```python
from build123d import *

# Parameters (mm, degrees)
F0_W     = 112
F0_H     = 30
F0_R     = 4
F1_DEPTH = 3
F3_DEPTH = 25
F4_R     = 4
F5_DEPTH = 25


with BuildPart() as f1:
    # F0 (on Front) → F1 (new body)
    with BuildSketch(Plane.XZ):
        Rectangle(F0_W, F0_H)
        with Locations((-45.5, 8)):
            Circle(F0_R, mode=Mode.SUBTRACT)
    extrude(amount=F1_DEPTH)

    # F2 (on face) → F3 (cut)
    with BuildSketch(Plane.XZ.offset(3)):
        Polygon((-39, 5), (-39, 2), (-39, -1), (-32, -1), (-32, -8), (-29, -8), (-26, -8), (-26, -1), (-19, -1), (-19, 2), (-19, 5), (-26, 5), (-26, 12), (-29, 12), (-32, 12), (-32, 5), align=None)
    extrude(amount=-F3_DEPTH, mode=Mode.SUBTRACT)

    # F4 (on face) → F5 (cut)
    with BuildSketch(Plane.XZ.offset(3)):
        with Locations((30.1, 0)):
            Circle(F4_R)
        with BuildLine():
            ThreePointArc((44.25, 0), (40.25, 4), (36.25, 0))
            ThreePointArc((36.25, 0), (40.25, -4), (44.25, 0))
        make_face()
    extrude(amount=-F5_DEPTH, mode=Mode.SUBTRACT)


solid = f1.part
```
Geometry: final body of the model. Coordinates: model frame, mm. A direction names the side the tool comes from. Coordinates: 2 decimals unless noted, no trailing zeros. Order: outer loops, then holes, each group sorted by start corner. A loop starts at its lowest first (then second) coordinate and runs counter-clockwise, first axis right, second up. Notation, with made-up numbers: M -19,32.5 L 9,32.5 A16 cw 9,45.5 Z; hole C 12,81 d1. An arc over 180 degrees is marked long. Answer in a Markdown table with one row per item. Add a question column.
Q1. Mould query, pull axis Z, two halves, no side actions, for faces 1 (the flat face through (-1, -1, 15)), 2 (the flat face through (-19, -2, 2)), 3 (the flat face through (56, -1, 0)). Classes: released by +Z, released by -Z, zero draft, split by the parting line, or undercut.
Q2. Section query C-C on y = -2. Return the cut outline in (x, z).
Q3. Reachability of faces 4 (the flat face through (-39, -2, 2)), 5 (the flat face through (-1, -1, -15)) from +Z, -Z, +X, -X, +Y, -Y: full face, straight path, thin tool, end or side. Return the list, or none.
Q4. Section query B-B on z = 8. Return the cut outline in (x, y).
Q5. Section query A-A on z = 0. Return the cut outline in (x, y).
Q6. Section query D-D on x = -45.5. Return the cut outline in (y, z), and give its area (3 significant figures).
Q7. Line query: L1, parallel to X at y = -2.8, z = 0.25; L2, parallel to X at y = -1.95, z = -7; L3, parallel to Z at x = -45.5, y = -1.35. Output: solid intervals per line, ascending.
Q8. Contact query for a flat-ended pin moving along its axis: P1, Ø6.5, axis at x = 40.25, z = 0, coming from the -Y side. Output: stop coordinate, or through.
Completed:
| question | item | result |
|---|---|---|
| 1 | face 1 | released by +Z |
| 1 | face 2 | undercut |
| 1 | face 3 | zero draft |
| 2 | outline | M -56,-15 L 56,-15 L 56,15 L -56,15 Z; hole C -45.5,8 d8; hole M -39,-1 L -32,-1 L -32,-8 L -26,-8 L -26,-1 L -19,-1 L -19,5 L -26,5 L -26,12 L -32,12 L -32,5 L -39,5 Z; hole C 30.1,0 d8; hole C 40.25,0 d8 |
| 3 | face 4 | +Y, -Y |
| 3 | face 5 | -Z, +X, -X, +Y, -Y |
| 4 | outline | M -56,-3 L -49.5,-3 L -49.5,0 L -56,0 Z; M -41.5,-3 L -32,-3 L -32,0 L -41.5,0 Z; M -26,-3 L 56,-3 L 56,0 L -26,0 Z |
| 5 | outline | M -56,-3 L -39,-3 L -39,0 L -56,0 Z; M -19,-3 L 26.1,-3 L 26.1,0 L -19,0 Z; M 34.1,-3 L 36.25,-3 L 36.25,0 L 34.1,0 Z; M 44.25,-3 L 56,-3 L 56,0 L 44.25,0 Z |
| 6 | outline | M -3,-15 L 0,-15 L 0,4 L -3,4 Z; M -3,12 L 0,12 L 0,15 L -3,15 Z |
| 6 | area | 66.0 mm2 |
| 7 | L1 | x = -56 to -39, -19 to 26.11, 34.09 to 36.26, 44.24 to 56 |
| 7 | L2 | x = -56 to -32, -26 to 56 |
| 7 | L3 | z = -15 to 4, 12 to 15 |
| 8 | P1 | passes through |
